Could you check a few things on this model? Use its own coordinates, in mm. A direction names the side the tool comes from. Coordinates: 2 decimals unless noted, no trailing zeros. Order: outer loops, then holes, each group sorted by start corner. A loop starts at its lowest first (then second) coordinate and runs counter-clockwise, first axis right, second up. Notation, with made-up numbers: (35, -5.75) - (52, -5.75) arc R14 cw to (52, 20.25) - close; hole circle Ø2 at (85.5, 57.5). An arc over 180 degrees is marked (long way). Answer as CSV lines item,"result". Start each with the question number.
1. I want a section at D-D, the plane x = 45. List the corners of the cut face in (y, z) for me.
2. Thinking about a two-plate mould opening in Z: for faces 1 (the face through (35, 2, -2)), 2 (the face through (48, 2, -15)), 3 (the face through (3, 2, -50)), which applies, released by +Z, released by -Z, zero draft, split by the parting line, or undercut?
3. I want a section at A-A, the plane z = -75. List the corners of the cut face in (x, y) for me.
4. For pin 1 (0.9 mm diameter, centred on y = 2, z = -6, fed in from +X); pin 2 (0.9 mm diameter, centred on x = 49, y = 2, fed in from -Z); pin 3 (0.9 mm diameter, centred on x = 48.5, y = 2, fed in from +Z), each with a flat end and sliding along its axis, tell me the tip position at first contact or that it passes through.
5. I need wall thicknesses on probe 1 along Z at (x, y) = (19.5, 2.55); probe 2 along Z at (x, y) = (45, 1.55); probe 3 along Z at (x, y) = (22.5, 2.75). Which ranges of each line are inside material? Lowest first, please.
6. I want a section at C-C, the plane y = 0.75. Count the separate pieces of the cut face and the enclosed holes in it, and give its area (3 significant figures).
7. For faces 4 (the face through (41, 2, -97)), 5 (the face through (41, 2, -3)), 6 (the face through (1, 2, -35)), 7 (the face through (49, 2, -35)), 8 (the face through (15, 2, -2)), which set-ups out of +Z, -Z, +X, -X, +Y, -Y let a thin tool reach every point of the face, with its end or its side?
8. I want a section at B-B, the plane x = 20. List the corners of the cut face in (y, z) for me, and give its area (3 significant figures).
Autodesk Inventor part; units mm, degrees
ref_plane "YZ Plane" through (0, 0, 0) normal (1, 0, 0) x (0, 1, 0)
ref_plane "XZ Plane" through (0, 0, 0) normal (0, 1, 0) x (-1, 0, 0)
ref_plane "XY Plane" through (0, 0, 0) normal (0, 0, 1) x (1, 0, 0)
sketch "Sketch1" plane through (0, 0, 0) normal (0, 1, 0) x (-1, 0, 0)
  line L0 (0, 0) -> (-50, 0)
  line L1 (-50, 0) -> (-50, -100)
  line L2 (-50, -100) -> (0, -100)
  line L3 (0, -100) -> (0, 0)
  dimension "d0" = 100
  dimension "d1" = 50
extrude "Base" add sketch "Sketch1" along normal blind 3
sketch "Sketch2" plane through (0, 3, 0) normal (0, 1, 0) x (1, 0, 0)
  line L0 (0, 0) -> (50, 0)
  line L1 (50, 100) -> (0, 100)
  line L2 (0, 0) -> (3, 0)
  line L3 (3, 100) -> (0, 100)
  line L4 (0, 100) -> (0, 0)
  line L5 (0, 100) -> (0, 0)
  line L6 (0, 0) -> (3, 0)
  line L7 (3, 0) -> (3, 15)
  line L8 (3, 15) -> (0, 15)
  line L9 (0, 15) -> (0, 0)
  line L10 (0, 100) -> (3, 100)
  line L11 (3, 100) -> (3, 85)
  line L12 (3, 85) -> (0, 85)
  line L13 (0, 85) -> (0, 100)
  line L14 (0, 35) -> (3, 35)
  line L15 (3, 35) -> (3, 65)
  line L16 (3, 65) -> (0, 65)
  line L17 (0, 65) -> (0, 35)
  line L18 (25, 0) -> (25, 100) construction
  line L19 (50, 0) -> (47, 0)
  line L20 (47, 100) -> (50, 100)
  line L21 (50, 100) -> (50, 0)
  line L22 (50, 100) -> (50, 0)
  line L23 (50, 0) -> (47, 0)
  line L24 (47, 0) -> (47, 15)
  line L25 (47, 15) -> (50, 15)
  line L26 (50, 15) -> (50, 0)
  line L27 (50, 100) -> (47, 100)
  line L28 (47, 100) -> (47, 85)
  line L29 (47, 85) -> (50, 85)
  line L30 (50, 85) -> (50, 100)
  line L31 (50, 35) -> (47, 35)
  line L32 (47, 35) -> (47, 65)
  line L33 (47, 65) -> (50, 65)
  line L34 (50, 65) -> (50, 35)
  line L35 (0, 50) -> (50, 50) construction
  line L36 (50, 0) -> (50, 100)
  line L37 (15, 0) -> (3, 0)
  line L38 (3, 0) -> (3, 3)
  line L39 (3, 3) -> (15, 3)
  line L40 (15, 3) -> (15, 0)
  line L41 (50, 0) -> (0, 0)
  line L42 (35, 0) -> (47, 0)
  line L43 (47, 3) -> (35, 3)
  line L44 (35, 3) -> (35, 0)
  line L45 (0, 100) -> (50, 100)
  line L46 (25, 100) -> (25, 0) construction
  line L47 (15, 100) -> (3, 100)
  line L48 (3, 97) -> (15, 97)
  line L49 (15, 97) -> (15, 100)
  line L50 (50, 100) -> (0, 100)
  line L51 (47, 97) -> (35, 97)
  line L52 (35, 100) -> (47, 100)
  line L53 (35, 97) -> (35, 100)
  point P0 (0, 15)
  point P1 (0, 85)
  point P2 (0, 65)
  point P3 (0, 35)
  point P4 (50, 100)
  point P5 (47, 97)
  point P6 (15, 100)
  point P7 (3, 97)
  dimension "d10" = 15
  dimension "d11" = 15
  dimension "d12" = 20
  dimension "d13" = 20
  dimension "d14" = 30
  dimension "d15" = 3
  dimension "d21" = 3
  dimension "d22" = 10
  dimension "d39" = 20
extrude "Tabs" cut sketch "Sketch2" against normal through all contours L4 L8 L7 L0 | L7 L39 L40 L0 | L4 L16 L15 L14 | L44 L43 L24 L0 | L24 L25 L21 L0 | L4 L1 L11 L12 | L1 L49 L48 L11 | L31 L32 L33 L21 | L1 L28 L51 L53 | L29 L28 L1 L21
sketch "Sketch4" plane through (0, 0, 0) normal (0, -1, 0) x (1, 0, 0)
  circle A0 centre (20, -46.603) radius 7.5
  circle A1 centre (20, -75) radius 7.5
  line L0 (50, -100) -> (0, -100)
  line L1 (3, -85) -> (3, -97)
  line L2 (3, -35) -> (3, -65)
  point P0 (0, 0)
  point P1 (35, -100)
  point P2 (15, -100)
  dimension "d31" = 25
  dimension "d32" = 28.397
  dimension "d33" = 17
  dimension "d34" = 17
  dimension "d35" = 15
  dimension "d36" = 15
extrude "BNC" cut sketch "Sketch4" against normal through all
equation "\"d0\" = Width"
equation "\"d2\" = Thickness"
equation "\"d10\" = WidthTabOffset"
equation "\"d11\" = d10"
equation "\"d12\" = BaseTabWidth"
equation "\"d13\" = d12"
equation "\"d15\" = Thickness"
equation "\"d21\" = d15"
equation "\"d22\" = 0.5 * VerticalTab"
equation "\"d34\" = d33"
equation "\"d36\" = d35"
properties part number "ShortSideFront"
Solved:
1,outline,"(0, -97) - (3, -97) - (3, -3) - (0, -3) - close"
2,face 1,"zero draft"
2,face 2,"released by +Z"
2,face 3,"undercut"
3,outline,"(0, 0) - (12.5, 0) - (12.5, 3) - (0, 3) - close; (27.5, 0) - (50, 0) - (50, 3) - (27.5, 3) - close"
4,pin 1,"stops at x = 47"
4,pin 2,"stops at z = -85"
4,pin 3,"stops at z = -15"
5,probe 1,"z = -100 to -82.48, -67.52 to -54.09, -39.12 to 0"
5,probe 2,"z = -97 to -3"
5,probe 3,"z = -100 to -82.07, -67.93 to -53.67, -39.53 to 0"
6,separate pieces,"1"
6,enclosed holes,"2"
6,area,"4,140 mm2"
7,face 4,"-Z, +X, +Y, -Y"
7,face 5,"+Z, +X, +Y, -Y"
7,face 6,"-X, +Y, -Y"
7,face 7,"+X, +Y, -Y"
7,face 8,"+Z, -X, +Y, -Y"
8,outline,"(0, -100) - (3, -100) - (3, -82.5) - (0, -82.5) - close; (0, -67.5) - (3, -67.5) - (3, -54.1) - (0, -54.1) - close; (0, -39.1) - (3, -39.1) - (3, 0) - (0, 0) - close"
8,area,"210 mm2"
